Check sheet for the modelled part. Datum: model origin and axes. Units: mm. Face numbers are marked on the shaded views. A direction names the side the tool comes from. Give positions to 0.01 mm unless a question says otherwise; leave off trailing zeros. Loops run counter-clockwise (first coordinate to the right, second up) from the corner with the lowest first, then second, coordinate; pieces in that order, holes last. Notation, with made-up numbers: (38, -14) -> (67, -14) arc R15 cw to (67, -8) -> close; hole circle Ø8 at (81, -18.75). An arc over 180 degrees is marked (long way). Write each question's results on one line, items separated by ' | '. Start each with the question number.
Item 1: Scan lines: line 1 along X through (y, z) = (-4.5, -0.75); line 2 along X through (y, z) = (1.5, -0.3); line 3 along Z through (x, y) = (0.25, -6). Record each from-to range of solid material in increasing order.
Item 2: Cross-section at A-A on y = 0. Enter the section's corners in (x, z), then the cut area to 3 significant figures.
Item 3: Mould release check, pull along Y, two halves, no side actions. Record for the marked faces 3, 4 and 5: pulls with the +Y half, pulls with the -Y half, needs draft (parallel to the pull), parting line crosses it, or undercut.
Item 4: Access from +Z, -Z, +X, -X, +Y, -Y to the whole of each face (thin tool, end or side, straight path). Record for the marked faces 1 and 2.
Item 5: Cross-section at D-D on y = 4. Enter the section's corners in (x, z), then the cut area to 3 significant figures.
Item 6: Cross-section at C-C on z = -0.4. State how many separate pieces and enclosed holes the cut face has, then the cut area to 3 significant figures.
Item 7: Gauge pin test, flat ends, axial feed: pin 1 Ø1.5 at (x, y) = (0, -6) entering from +Z; pin 2 Ø2 at (x, y) = (-4.5, -1.5) entering from -Z. Record the tip position at first contact, or that the pin passes through.
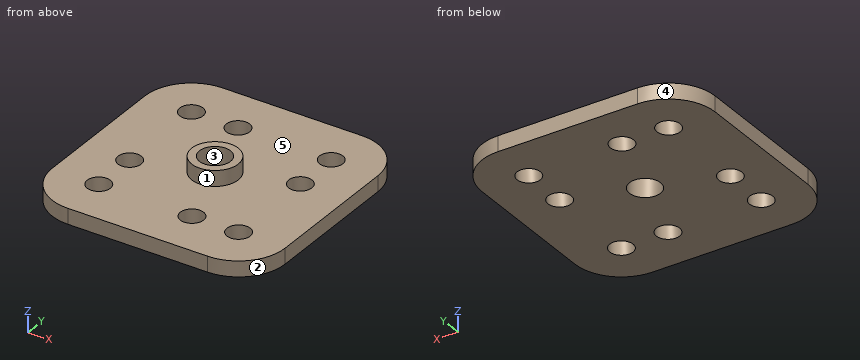
from build123d import *

# Parameters (mm, degrees)
F0_R            = 1.5
F0_R_2          = 1
F1_DEPTH        = 1
F2_W            = 15
F2_H            = 15
F2_R            = 5
F2_R_2          = 1.5
F2_R_3          = 1
F3_DEPTH        = 1
F4_R            = 3
F5_R            = 0.75
F6_DEPTH        = 25
F6_COPIES_COUNT = 4


# Not quite as in the source:
# - a pattern or mirror of a feature is missing from the dataset's text; its kind, count and spacing are read off the source's solid


with BuildPart() as f1:
    # F0 (on Top) → F1 (new body)
    with BuildSketch(Plane.XY):
        Circle(F0_R)
        Circle(F0_R_2, mode=Mode.SUBTRACT)
    extrude(amount=F1_DEPTH)

    # F2 (on face) → F3 (join)
    with BuildSketch(Plane(origin=(0, 0, 0), x_dir=(1, 0, 0), z_dir=(0, 0, -1))):
        Rectangle(F2_W, F2_H)
        Circle(F2_R, mode=Mode.SUBTRACT)
        Circle(F2_R)
        Circle(F2_R_2, mode=Mode.SUBTRACT)
        Circle(F2_R_2)
        Circle(F2_R_3, mode=Mode.SUBTRACT)
    extrude(amount=F3_DEPTH)

    # F4
    f4_edges = [f1.edges().sort_by_distance(p)[0] for p in [
        (-7.5, 7.5, -0.5),
        (7.5, 7.5, -0.5),
        (-7.5, -7.5, -0.5),
        (7.5, -7.5, -0.5),
    ]]
    fillet(f4_edges, radius=F4_R)

    # F5 (on face) → F6 (cut)
    with BuildSketch(Plane.XY):
        with Locations((-4.5, 4.5)):
            Circle(F5_R)
        with Locations((-1.5, 4.5)):
            Circle(F5_R)
    f6 = extrude(amount=-F6_DEPTH, mode=Mode.SUBTRACT)

    # F6_copies: F6 ×4 about axis
    f6_copies_axis = Axis((0, 0, 0), (0, 0, 1))
    for i in range(1, F6_COPIES_COUNT):
        add(f6.rotate(f6_copies_axis, i * 360 / F6_COPIES_COUNT), mode=Mode.SUBTRACT)


solid = f1.part
Answer sheet:
1) line 1: x = -7.5 to -5.25, -3.75 to 0.75, 2.25 to 3.75, 5.25 to 7.5 | line 2: x = -7.5 to 3.75, 5.25 to 7.5 | line 3: z = -1 to 0
2) outline: (-7.5, -1) -> (-1, -1) -> (-1, 1) -> (-1.5, 1) -> (-1.5, 0) -> (-7.5, 0) -> close; (1, -1) -> (7.5, -1) -> (7.5, 0) -> (1.5, 0) -> (1.5, 1) -> (1, 1) -> close | area: 14.0 mm²
3) face 3: undercut | face 4: pulls with the +Y half | face 5: needs draft
4) face 1: +Z | face 2: +Z, -Z, +X, -Y
5) outline: (-7.5, -1) -> (-5.06, -1) -> (-5.06, 0) -> (-7.5, 0) -> close; (-3.94, -1) -> (-2.06, -1) -> (-2.06, 0) -> (-3.94, 0) -> close; (-0.94, -1) -> (3.94, -1) -> (3.94, 0) -> (-0.94, 0) -> close; (5.06, -1) -> (7.5, -1) -> (7.5, 0) -> (5.06, 0) -> close | area: 11.6 mm²
6) separate pieces: 1 | enclosed holes: 9 | area: 200 mm²
7) pin 1: stops at z = 0 | pin 2: stops at z = -1
